```python
from build123d import *

# Parameters (mm, degrees)
SKETCH1_R           = 265.7
SKETCH1_R_2         = 211.5
SKETCH1_R_3         = 20
SKETCH1_R_4         = 5
EXTRUDE1_DEPTH      = 5
SKETCH2_R           = 265.7
SKETCH2_R_2         = 15
SKETCH2_R_3         = 211.5
EXTRUDE2_DEPTH      = 25
SKETCH3_R           = 265.7
SKETCH3_R_2         = 260.7
EXTRUDE3_DEPTH      = 200
SKETCH4_R           = 102.37
EXTRUDE4_DEPTH      = 266.7
SKETCH5_R           = 117.4
EXTRUDE5_DEPTH      = 266.7000001
SKETCH6_W           = 200
SKETCH6_H           = 79
EXTRUDE6_DEPTH      = 266.7000001
EXTRUDE6_DEPTH_BACK = 266.7000001


with BuildPart() as part:
    # Sketch1 → Extrude1 (new body)
    with BuildSketch(Plane.XY):
        Circle(SKETCH1_R)
        Circle(SKETCH1_R_2, mode=Mode.SUBTRACT)
        with Locations((238.6, 0)):
            Circle(SKETCH1_R_3, mode=Mode.SUBTRACT)
        with Locations((168.715677991, 168.715677991)):
            Circle(SKETCH1_R_3, mode=Mode.SUBTRACT)
        with Locations((0, 238.6)):
            Circle(SKETCH1_R_3, mode=Mode.SUBTRACT)
        with Locations((-168.715677991, 168.715677991)):
            Circle(SKETCH1_R_3, mode=Mode.SUBTRACT)
        with Locations((-238.6, 0)):
            Circle(SKETCH1_R_3, mode=Mode.SUBTRACT)
        with Locations((-168.715677991, -168.715677991)):
            Circle(SKETCH1_R_3, mode=Mode.SUBTRACT)
        with Locations((0, -238.6)):
            Circle(SKETCH1_R_3, mode=Mode.SUBTRACT)
        with Locations((168.715677991, -168.715677991)):
            Circle(SKETCH1_R_3, mode=Mode.SUBTRACT)
        with Locations((230.469902153, 61.754224161)):
            Circle(SKETCH1_R_4, mode=Mode.SUBTRACT)
        with Locations((-230.469902153, 61.754224161)):
            Circle(SKETCH1_R_4, mode=Mode.SUBTRACT)
        with Locations((-91.308266962, -220.437656457)):
            Circle(SKETCH1_R_4, mode=Mode.SUBTRACT)
    extrude(amount=EXTRUDE1_DEPTH)

    # Sketch2 → Extrude2 (add)
    with BuildSketch(Plane.XY.offset(5)):
        Circle(SKETCH2_R)
        with Locations((238.6, 0)):
            Circle(SKETCH2_R_2, mode=Mode.SUBTRACT)
        with Locations((168.715677991, 168.715677991)):
            Circle(SKETCH2_R_2, mode=Mode.SUBTRACT)
        with Locations((0, 238.6)):
            Circle(SKETCH2_R_2, mode=Mode.SUBTRACT)
        with Locations((-168.715677991, 168.715677991)):
            Circle(SKETCH2_R_2, mode=Mode.SUBTRACT)
        with Locations((-238.6, 0)):
            Circle(SKETCH2_R_2, mode=Mode.SUBTRACT)
        with Locations((-168.715677991, -168.715677991)):
            Circle(SKETCH2_R_2, mode=Mode.SUBTRACT)
        with Locations((0, -238.6)):
            Circle(SKETCH2_R_2, mode=Mode.SUBTRACT)
        with Locations((168.715677991, -168.715677991)):
            Circle(SKETCH2_R_2, mode=Mode.SUBTRACT)
        Circle(SKETCH2_R_3, mode=Mode.SUBTRACT)
    extrude(amount=EXTRUDE2_DEPTH)

    # Sketch3 → Extrude3 (add)
    with BuildSketch(Plane.XY.offset(30)):
        Circle(SKETCH3_R)
        Circle(SKETCH3_R_2, mode=Mode.SUBTRACT)
    extrude(amount=EXTRUDE3_DEPTH)

    # Sketch4 → Extrude4 (cut, through all)
    with BuildSketch(Plane(origin=(0, 0, 0), x_dir=(0, 0, -1), z_dir=(1, 0, 0))):
        with Locations((-250, 0)):
            Circle(SKETCH4_R)
    extrude(amount=EXTRUDE4_DEPTH, mode=Mode.SUBTRACT)

    # Sketch5 → Extrude5 (cut, through all)
    with BuildSketch(Plane(origin=(0, 0, 0), x_dir=(0, 0, -1), z_dir=(1, 0, 0))):
        with Locations((-250, 0)):
            Circle(SKETCH5_R)
    extrude(amount=-EXTRUDE5_DEPTH, mode=Mode.SUBTRACT)

    # Sketch6 → Extrude6 (cut, two sides)
    with BuildSketch(Plane(origin=(0, 0, 0), x_dir=(1, 0, 0), z_dir=(0, 1, 0))) as extrude6_sk:
        with Locations((0, -190.5)):
            Rectangle(SKETCH6_W, SKETCH6_H)
    extrude(amount=EXTRUDE6_DEPTH, mode=Mode.SUBTRACT)
    extrude(extrude6_sk.sketch, amount=-EXTRUDE6_DEPTH_BACK, mode=Mode.SUBTRACT)


solid = part.part
```
For this review, take the finished solid that the model builds, in its own axes (mm). A direction names the side the tool comes from. Round coordinates to 2 decimals unless told otherwise and drop trailing zeros. Write each loop counter-clockwise with the first axis right and the second up, starting at its lowest first coordinate (ties: lowest second). Pieces come first, ordered by that corner, then holes.
1) Take a section at D-D on z = 204.5. Give the boundary of the cut face in (x, y) (3 decimals), then the cut area to 3 significant figures.
Answer below:
outline: (-242.66, -108.224) arc R265.7 ccw to (-100, -246.164) - (-100, -240.758) arc R260.7 cw to (-237.175, -108.224) - close; (-242.66, 108.224) - (-237.175, 108.224) arc R260.7 cw to (-100, 240.758) - (-100, 246.164) arc R265.7 ccw to start; (100, -246.164) arc R265.7 ccw to (249.373, -91.703) - (244.039, -91.703) arc R260.7 cw to (100, -240.758) - close; (100, 240.758) arc R260.7 cw to (244.039, 91.703) - (249.373, 91.703) arc R265.7 ccw to (100, 246.164) - close
area: 4,170 mm2
2) Mouldability with a two-part tool opening along Y and no side actions: class faces 1 (the face through (183, 190, 230)), 2 (the face through (-4.336, -258.124, 2.465)) as +Y half, -Y half, draft (parallel to the pull), parting line (faces both ways), or undercut.
Answer below:
face 1: draft
face 2: undercut
3) For line 1 along Y through (x, z) = (0, 1.2); line 2 along X through (y, z) = (100.5, 73.5); line 3 along X through (y, z) = (-17.5, 80), list the stretches that pass through material, from the lowest coordinate up.
Answer below:
line 1: y = -265.7 to -258.6, -218.6 to -211.5, 211.5 to 218.6, 258.6 to 265.7
line 2: x = -245.96 to -240.55, 240.55 to 245.96
line 3: x = -265.12 to -260.11, 260.11 to 265.12
4) Insertion check: pin 1 Ø6 at (x, y) = (-91.31, -220.44) entering from +Z; pin 2 Ø1.5 at (y, z) = (-112.5, 44) entering from +X; pin 3 Ø1 at (y, z) = (-208, 161.5) entering from +X. Each pin has a flat end and moves straight along its axis. Give the tip position at first contact, or say it passes through.
Answer below:
pin 1: stops at z = 30
pin 2: stops at x = 241.06
pin 3: stops at x = 165.95
5) Take a section at B-B on z = 174. Give the boundary of the cut face in (x, y).
Answer below:
outline: (-250.18, -89.48) arc R265.7 ccw to (-100, -246.16) - (-100, -240.76) arc R260.7 cw to (-244.86, -89.48) - close; (-250.18, 89.48) - (-244.86, 89.48) arc R260.7 cw to (-100, 240.76) - (-100, 246.16) arc R265.7 ccw to start; (100, -246.16) arc R265.7 ccw to (256.7, -68.58) - (251.52, -68.58) arc R260.7 cw to (100, -240.76) - close; (100, 240.76) arc R260.7 cw to (251.52, 68.58) - (256.7, 68.58) arc R265.7 ccw to (100, 246.16) - close
6) Machinability: for faces 3 (the face through (-180, 191, 230)), 4 (the face through (-157.964, -151.852, 2.465)), 5 (the face through (-261.475, -0.767, 132.603)), which of the approach directions +Z, -Z, +X, -X, +Y, -Y give a long, thin tool a straight path to every point of the face, cutting with its end or side? Answer none if there is none.
Answer below:
face 3: +Z, +X, -X, +Y, -Y
face 4: -Z
face 5: +Z, -X
7) Take a section at A-A on x = 136. Give the boundary of the cut face in (y, z).
Answer below:
outline: (-228.26, 0) - (-161.98, 0) - (-161.98, 30) - (-222.42, 30) - (-222.42, 230) - (-228.26, 230) - close; (161.98, 0) - (228.26, 0) - (228.26, 230) - (222.42, 230) - (222.42, 30) - (161.98, 30) - close
8) Take a section at C-C on y = 141.5. Give the boundary of the cut face in (x, z).
Answer below:
outline: (-224.89, 0) - (-157.19, 0) - (-157.19, 30) - (-218.96, 30) - (-218.96, 230) - (-224.89, 230) - close; (157.19, 0) - (224.89, 0) - (224.89, 230) - (218.96, 230) - (218.96, 30) - (157.19, 30) - close
